Build history of the part. All positions in model axes, mm. Round coordinates to 2 decimals unless told otherwise and drop trailing zeros. Loops run counter-clockwise (first coordinate to the right, second up) from the corner with the lowest first, then second, coordinate; pieces in that order, holes last. Notation, with made-up numbers: M 26.5,30 L 64.5,30 A18 ccw 64.5,41 Z; hole C 36,82 d4. An arc over 180 degrees is marked long. One line per item, written item: value.
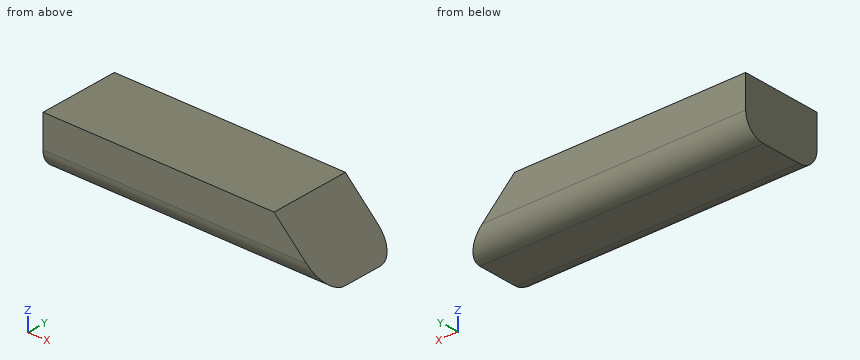
```python
from build123d import *

# Parameters (mm, degrees)
BOSS_EXTRUDE1_DEPTH = 444.5
SKETCH2_W           = 344.402501539
SKETCH2_H           = 780.457540958
CUT_EXTRUDE1_DEPTH  = 59.371664787


with BuildPart() as part:
    # Sketch1 → Boss-Extrude1 (new body)
    with BuildSketch(Plane(origin=(0, 0, 0), x_dir=(0, 0, -1), z_dir=(1, 0, 0))):
        with BuildLine():
            Line((0, 0), (31.75, 0))
            ThreePointArc((31.75, 0), (54.200640303, 9.299359697), (63.5, 31.75))
            Line((63.5, 31.75), (63.5, 95.25))
            ThreePointArc((63.5, 95.25), (54.200640303, 117.700640303), (31.75, 127))
            Line((31.75, 127), (0, 127))
            Line((0, 127), (-19.05, 127))
            Line((-19.05, 127), (-19.05, 0))
            Line((-19.05, 0), (0, 0))
        make_face()
    extrude(amount=BOSS_EXTRUDE1_DEPTH)

    # Sketch2 → Cut-Extrude1 (cut, through all)
    with BuildSketch(Plane(origin=(190.5, 0, 190.5), x_dir=(0, 1, 0), z_dir=(0.707106781, 0, 0.707106781))):
        with Locations((32.995160032, -359.210244843)):
            Rectangle(SKETCH2_W, SKETCH2_H)
    extrude(amount=CUT_EXTRUDE1_DEPTH, mode=Mode.SUBTRACT)


solid = part.part
```
Item 1: Slice it at C-C, the plane y = 52. Give the cut face in (x, z).
Check values:
outline: M 0,-63.5 L 444.5,-63.5 L 361.95,19.05 L 0,19.05 Z
Item 2: Slice it at A-A, the plane x = 125. Give the cut face in (y, z), and give its area (3 significant figures).
Check values:
outline: M 0,-31.75 A31.75 ccw 31.75,-63.5 L 95.25,-63.5 A31.75 ccw 127,-31.75 L 127,19.05 L 0,19.05 Z
area: 10,100 mm2
Item 3: Slice it at B-B, the plane z = 0.5. Give the cut face in (x, y).
Check values:
outline: M 0,0 L 380.5,0 L 380.5,127 L 0,127 Z
Item 4: Wall check: line 1 along Y through (x, z) = (402.5, -43.5); line 2 along Y through (x, z) = (32.5, -32.5); line 3 along X through (y, z) = (21, -29.5). Give the ranges that are in metal, low to high.
Check values:
line 1: y = 2.25 to 124.75
line 2: y = 0.01 to 126.99
line 3: x = 0 to 410.5
